Autodesk Fusion 360 part; units mm, degrees
sketch "Sketch1" plane through (0, 0, 0) normal (1, 0, 0) x (0, 1, 0)
  line L0 (0, 0) -> (0, -15)
  line L1 (0, -15) -> (30, -15)
  line L2 (30, -15) -> (45.75, -15)
  line L3 (60.75, -15) -> (60.75, -22.5)
  line L4 (60.75, -37.5) -> (82.75, -37.5)
  line L5 (82.75, -37.5) -> (82.75, -22.5)
  line L6 (60.75, 0) -> (0, 0)
  line L7 (45.75, -15) -> (45.75, -37.5)
  line L8 (45.75, -37.5) -> (60.75, -37.5)
  line L9 (60.75, 0) -> (60.75, -15)
  line L10 (60.75, -22.5) -> (82.75, -22.5)
  dimension "d1" = 15
  dimension "d2" = 30
  dimension "d3" = 30.75
  dimension "d4" = 22.5
  dimension "d5" = 22
  dimension "d6" = 15
  dimension "d8" = 15
  dimension "d9" = 15
extrude "Extrude1" add sketch "Sketch1" along normal blind 40
sketch "Sketch2" plane through (0, 0, -22.5) normal (0, 0, 1) x (-1, 0, 0)
  line L0 (0, -82.75) -> (0, -60.75)
  line L1 (0, -60.75) -> (-40, -60.75)
  line L2 (-40, -60.75) -> (-40, -82.75)
  line L3 (-40, -82.75) -> (0, -82.75)
  line L4 (-40, -82.75) -> (-34.9, -82.75) construction
  line L5 (-20, -82.75) -> (-20, -60.75) construction
  line L6 (-20, -77.95) -> (-5.5, -77.95) construction
  circle A0 centre (-5.5, -77.95) radius 1.6
  circle A1 centre (-5.5, -71.95) radius 1.6
  circle A2 centre (-5.5, -65.95) radius 1.6
  circle A3 centre (-34.5, -77.95) radius 1.6
  circle A4 centre (-34.5, -71.95) radius 1.6
  circle A5 centre (-34.5, -65.95) radius 1.6
  dimension "d40" = 3.2
  dimension "d41" = 3.2
  dimension "d42" = 3.2
fillet "Fillet1" radius 2 8 edges at (20, 0, 0) (20, 0, -15) (20, 60.75, 0) (20, 60.75, -22.5) (20, 82.75, -22.5) (20, 82.75, -37.5) (20, 45.75, -37.5) (20, 45.75, -15)
fillet "Fillet2" radius 2 16 edges at (40, 0.5858, -0.5858) (40, 0, -7.5) (40, 0.5858, -14.4142) (40, 22.875, -15) (40, 45.1642, -15.5858) (40, 45.75, -26.25) (40, 46.3358, -36.9142) (40, 64.25, -37.5) (40, 82.1642, -36.9142) (40, 82.75, -30) (40, 82.1642, -23.0858) (40, 71.75, -22.5) (40, 61.3358, -21.9142) (40, 60.75, -11.25) (40, 60.1642, -0.5858) (40, 30.375, 0)
sketch "Sketch3" plane through (0, 0, 0) normal (0, 0, 1) x (-1, 0, 0)
  line L0 (-38, -2) -> (-38, -58.75)
  line L1 (-38, -58.75) -> (0, -58.75)
  line L2 (0, -58.75) -> (0, -2)
  line L3 (0, -2) -> (-38, -2)
  circle A0 centre (-19, -11.5) radius 0.8
  line L4 (-19, -22) -> (-19, -14.5) construction
  circle A1 centre (-30.6913, -28.75) radius 0.8
  circle A2 centre (-12.5048, -25.75) radius 0.8
  circle A3 centre (-35.5, -22) radius 0.8
  circle A4 centre (-19, -5.5) radius 0.8
  circle A5 centre (-33.2894, -13.75) radius 0.8
  circle A6 centre (-19, -32.5) radius 0.8
  circle A7 centre (-28.0933, -27.25) radius 0.8
  circle A8 centre (-12.5048, -18.25) radius 0.8
  circle A9 centre (-32.5, -22) radius 0.8
  line L5 (-19, 19.2574) -> (-19, -41.0839) construction
  circle A10 centre (-25.4952, -18.25) radius 0.8
  circle A11 centre (-2.5, -22) radius 0.8
  line L6 (-19, -22) -> (-19, -5.5) construction
  circle A12 centre (-9.9067, -16.75) radius 0.8
  circle A13 centre (-30.6913, -15.25) radius 0.8
  circle A14 centre (-8.5, -22) radius 0.8
  circle A15 centre (-7.3087, -28.75) radius 0.8
  circle A16 centre (-28.0933, -16.75) radius 0.8
  circle A17 centre (-19, -38.5) radius 0.8
  line L7 (-19, -22) -> (-19, -8.5) construction
  circle A18 centre (-19, -29.5) radius 0.8
  line L8 (-19, -22) -> (-19, -11.5) construction
  circle A19 centre (-5.5, -22) radius 0.8
  circle A20 centre (-19, -35.5) radius 0.8
  circle A21 centre (-11.5, -22) radius 0.8
  circle A22 centre (-29.5, -22) radius 0.8
  circle A23 centre (-19, -22) radius 19
  circle A24 centre (-4.7106, -30.25) radius 0.8
  circle A25 centre (-33.2894, -30.25) radius 0.8
  circle A26 centre (-19, -14.5) radius 0.8
  circle A27 centre (-25.4952, -25.75) radius 0.8
  circle A28 centre (-9.9067, -27.25) radius 0.8
  circle A29 centre (-26.5, -22) radius 0.8
  circle A30 centre (-7.3087, -15.25) radius 0.8
  circle A31 centre (-4.7106, -13.75) radius 0.8
  circle A32 centre (-19, -8.5) radius 0.8
  line L9 (0, -2) -> (-19, -2) construction
  line L10 (-19, -2) -> (-19, -22) construction
  point P0 (-19, -22)
  dimension "d25" = 360
  dimension "d27" = 90
  dimension "d28" = 38
  dimension "d29" = 7.5
  dimension "d30" = 1.6
  dimension "d31" = 10.5
  dimension "d32" = 1.6
  dimension "d33" = 13.5
  dimension "d34" = 1.6
  dimension "d35" = 16.5
  dimension "d36" = 1.6
  dimension "d37" = 20
extrude "Extrude4" cut sketch "Sketch2" against normal through all contours A0 | A1 | A2 | A3 | A4 | A5
sketch "Sketch4" plane through (0, 0, 0) normal (0, 0, 1) x (-1, 0, 0)
  line L0 (-38, -2) -> (-38, -58.75)
  line L1 (-38, -58.75) -> (0, -58.75)
  line L2 (0, -58.75) -> (0, -2)
  line L3 (0, -2) -> (-38, -2)
  line L4 (-19, -2) -> (-19, -22) construction
  circle A0 centre (-19, -22) radius 19
  line L5 (-19, -22) -> (-19, -29) construction
  circle A1 centre (-19, -29) radius 1.6
  circle A2 centre (-12, -22) radius 1.6
  circle A3 centre (-19, -15) radius 1.6
  circle A4 centre (-26, -22) radius 1.6
  circle A5 centre (-19, -22) radius 3.5
  dimension "d44" = 20
  dimension "d45" = 38
  dimension "d46" = 7
  dimension "d47" = 3.2
  dimension "d49" = 360
  dimension "d50" = 7
extrude "Extrude5" cut sketch "Sketch4" against normal through all contours A1 | A2 | A3 | A4 | A5
equation "d29 = ( 15 / 2 ) * 1 mm"
equation "d31 = ( 21 / 2 ) * 1 mm"
equation "d33 = ( 27 / 2 ) * 1 mm"
equation "d35 = ( 33 / 2 ) * 1 mm"
equation "d46 = ( 14 / 2 ) * 1 mm"
Could you check a few things on this model? Use its own coordinates, in mm. A direction names the side the tool comes from. Round coordinates to 2 decimals unless told otherwise and drop trailing zeros. Write each loop counter-clockwise with the first axis right and the second up, starting at its lowest first coordinate (ties: lowest second). Pieces come first, ordered by that corner, then holes. Notation, with made-up numbers: (86, 20.5) -> (142, 20.5) arc R17 ccw to (142, 42.5) -> close; hole circle Ø11 at (41, 87.5). An arc over 180 degrees is marked (long way). Use a Markdown table: item, result.
1. We'd pull the mould along Y, two halves only. Please class faces 1 (the face through (19, 64, -37.5)), 2 (the face through (19.27, 82.15, -36.93)), 3 (the face through (34.708, 76.364, -29.895)): +Y half, -Y half, draft (parallel to the pull), parting line (faces both ways), or undercut.
Answer key:
| item | result |
|---|---|
| face 1 | draft |
| face 2 | +Y half |
| face 3 | undercut |
2. If we section it at D-D (z = -8.5): List the corners of the cut face in (x, y) for me.
Answer key:
| item | result |
|---|---|
| outline | (0, 0) -> (38, 0) arc R2 ccw to (40, 2) -> (40, 58.75) arc R2 ccw to (38, 60.75) -> (0, 60.75) -> close; hole circle Ø3.2 at (12, 22); hole circle Ø7 at (19, 22); hole circle Ø3.2 at (19, 15); hole circle Ø3.2 at (19, 29); hole circle Ø3.2 at (26, 22) |
3. If we section it at B-B (x = 5.5): List the corners of the cut face in (y, z) for me, then the cut area to 3 significant figures.
Answer key:
| item | result |
|---|---|
| outline | (0, -13) arc R2 ccw to (2, -15) -> (43.75, -15) arc R2 cw to (45.75, -17) -> (45.75, -35.5) arc R2 ccw to (47.75, -37.5) -> (64.35, -37.5) -> (64.35, -22.5) -> (62.75, -22.5) arc R2 cw to (60.75, -20.5) -> (60.75, -2) arc R2 ccw to (58.75, 0) -> (2, 0) arc R2 ccw to (0, -2) -> close; (67.55, -37.5) -> (70.35, -37.5) -> (70.35, -22.5) -> (67.55, -22.5) -> close; (73.55, -37.5) -> (76.35, -37.5) -> (76.35, -22.5) -> (73.55, -22.5) -> close; (79.55, -37.5) -> (80.75, -37.5) arc R2 ccw to (82.75, -35.5) -> (82.75, -24.5) arc R2 ccw to (80.75, -22.5) -> (79.55, -22.5) -> close |
| area | 1,430 mm^2 |
4. Which directions (+Z, -Z, +X, -X, +Y, -Y) give clear straight access to the entire face, cutting with the end or side of a thin tool? Please do faces 4 (the face through (39.43, 71.62, -23.1)), 5 (the face through (39.43, 46.35, -26.38)), 6 (the face through (15, 23, -15)).
Answer key:
| item | result |
|---|---|
| face 4 | +Z, +X, +Y |
| face 5 | -Z, +X, -Y |
| face 6 | -Z, +X, -X, -Y |
5. Please list where these lines run through material, in increasing order: probe 1 along Y at (x, z) = (5.5, -28); probe 2 along X at (y, z) = (77.95, -31.5); probe 3 along X at (y, z) = (22, -3).
Answer key:
| item | result |
|---|---|
| probe 1 | y = 45.75 to 64.35, 67.55 to 70.35, 73.55 to 76.35, 79.55 to 82.75 |
| probe 2 | x = 0 to 3.9, 7.1 to 32.9, 36.1 to 40 |
| probe 3 | x = 0 to 10.4, 13.6 to 15.5, 22.5 to 24.4, 27.6 to 40 |
6. For pin 1 Ø3.5 at (x, y) = (19, 15) entering from -Z; pin 2 Ø9 at (x, y) = (15, 68) entering from +Z; pin 3 Ø5.5 at (x, z) = (26.5, -10.5) entering from +Y, each with a flat end and sliding along its axis, tell me the tip position at first contact or that it passes through.
Answer key:
| item | result |
|---|---|
| pin 1 | stops at z = -15 |
| pin 2 | stops at z = -22.5 |
| pin 3 | stops at y = 60.75 |
7. If we section it at C-C (y = 65.95): List the corners of the cut face in (x, z) for me.
Answer key:
| item | result |
|---|---|
| outline | (0, -37.5) -> (3.9, -37.5) -> (3.9, -22.5) -> (0, -22.5) -> close; (7.1, -37.5) -> (32.9, -37.5) -> (32.9, -22.5) -> (7.1, -22.5) -> close; (36.1, -37.5) -> (38, -37.5) arc R2 ccw to (40, -35.5) -> (40, -24.5) arc R2 ccw to (38, -22.5) -> (36.1, -22.5) -> close |
8. If we section it at A-A (y = 22): List the corners of the cut face in (x, z) for me.
Answer key:
| item | result |
|---|---|
| outline | (0, -15) -> (10.4, -15) -> (10.4, 0) -> (0, 0) -> close; (13.6, -15) -> (15.5, -15) -> (15.5, 0) -> (13.6, 0) -> close; (22.5, -15) -> (24.4, -15) -> (24.4, 0) -> (22.5, 0) -> close; (27.6, -15) -> (38, -15) arc R2 ccw to (40, -13) -> (40, -2) arc R2 ccw to (38, 0) -> (27.6, 0) -> close |
